```python
from build123d import *

# Parameters (mm, degrees)
F0_R     = 20
F1_DEPTH = 2
F2_W     = 370
F2_H     = 270
F3_DEPTH = 12


with BuildPart() as f1:
    # F0 (on Top) → F1 (new body)
    with BuildSketch(Plane.XY):
        with Locations((0, 200)):
            Circle(F0_R)
        with Locations((75, 200)):
            Circle(F0_R)
        with Locations((150, 200)):
            Circle(F0_R)
        with Locations((225, 200)):
            Circle(F0_R)
        with Locations((300, 200)):
            Circle(F0_R)
        with Locations((262.5, 150)):
            Circle(F0_R)
        with Locations((300, 100)):
            Circle(F0_R)
        with Locations((300, 0)):
            Circle(F0_R)
        with Locations((187.5, 150)):
            Circle(F0_R)
        with Locations((112.5, 150)):
            Circle(F0_R)
        with Locations((37.5, 150)):
            Circle(F0_R)
        with BuildLine():
            ThreePointArc((12, 84), (17.888544, 91.055728), (20, 100))
            ThreePointArc((20, 100), (-17.888544, 108.944272), (12, 84))
        make_face()
        with Locations((75, 100)):
            Circle(F0_R)
        with Locations((150, 100)):
            Circle(F0_R)
        with Locations((225, 100)):
            Circle(F0_R)
        with Locations((262.5, 50)):
            Circle(F0_R)
        with Locations((187.5, 50)):
            Circle(F0_R)
        with Locations((225, 0)):
            Circle(F0_R)
        with Locations((150, 0)):
            Circle(F0_R)
        with Locations((112.5, 50)):
            Circle(F0_R)
        with BuildLine():
            ThreePointArc((57.5, 50), (46.444272, 67.888544), (25.5, 66))
            Line((25.5, 66), (49.5, 34))
            ThreePointArc((49.5, 34), (55.388544, 41.055728), (57.5, 50))
        make_face()
        Circle(F0_R)
        with BuildLine():
            ThreePointArc((95, 0), (83.944272, 17.888544), (63, 16))
            ThreePointArc((63, 16), (66.055728, -17.888544), (95, 0))
        make_face()
        with BuildLine():
            Line((49.5, 34), (25.5, 66))
            ThreePointArc((25.5, 66), (21.5, 38), (49.5, 34))
        make_face()
    extrude(amount=-F1_DEPTH)


with BuildPart() as f3:
    # F2 (on Top) → F3 (new body)
    with BuildSketch(Plane.XY):
        with Locations((150, 100)):
            Rectangle(F2_W, F2_H)
    extrude(amount=-F3_DEPTH)

    # F4: cut F1
    add(f1.part, mode=Mode.SUBTRACT)


solid = f3.part
```
CAD build for the part. Positions are in the model's coordinates, mm. Round coordinates to 2 decimals unless told otherwise and drop trailing zeros. Loops run counter-clockwise (first coordinate to the right, second up) from the corner with the lowest first, then second, coordinate; pieces in that order, holes last. Notation, with made-up numbers: M 83.25,80.5 L 126.25,80.5 A23 ccw 126.25,111.5 Z; hole C 72.25,84 d1. An arc over 180 degrees is marked long. Use a Markdown table: item, result. Add a question column.
(1) Drill centre lines: line 1 (Y direction, x = 75, z = -0.5); line 2 (Y direction, x = 125, z = -1); line 3 (Z direction, x = 46, y = 133.5). Where is each one in solid material? Low to high.
(2) Pull direction Y, two halves, no side cores. Call faces 1 (the face through (300, 0, -2)), 2 (the face through (0, 100, -2)), 3 (the face through (147, 235, -6)): +Y half, -Y half, draft (parallel to the pull), parting line (faces both ways), or undercut.
(3) Cut at A-A (x = 300). Give the cut face in (y, z), and give its area (3 significant figures).
(4) Cut at B-B (y = 6). Give the cut face in (x, z).
(5) Cut at C-C (x = 37.5). Give the cut face in (y, z).
(6) Cut at D-D (y = 164). Give the cut face in (x, z).
(7) Flat gauge pins, fed straight in: pin 1 (20 mm diameter, centred on x = 9, y = 208.5, fed in from +Z); pin 2 (20 mm diameter, centred on x = 302.5, y = 96, fed in from +Z). Where does each tip first touch, or does it go through?
Geometry says:
| question | item | result |
|---|---|---|
| 1 | line 1 | y = -35 to -20, 20 to 80, 120 to 180, 220 to 235 |
| 1 | line 2 | y = -35 to 34.39, 65.61 to 134.39, 165.61 to 235 |
| 1 | line 3 | z = -12 to -2 |
| 2 | face 1 | undercut |
| 2 | face 2 | undercut |
| 2 | face 3 | +Y half |
| 3 | outline | M -35,-12 L 235,-12 L 235,0 L 220,0 L 220,-2 L 180,-2 L 180,0 L 120,0 L 120,-2 L 80,-2 L 80,0 L 20,0 L 20,-2 L -20,-2 L -20,0 L -35,0 Z |
| 3 | area | 3,000 mm² |
| 4 | outline | M -35,-12 L 335,-12 L 335,0 L 319.08,0 L 319.08,-2 L 280.92,-2 L 280.92,0 L 244.08,0 L 244.08,-2 L 205.92,-2 L 205.92,0 L 169.08,0 L 169.08,-2 L 130.92,-2 L 130.92,0 L 94.08,0 L 94.08,-2 L 55.92,-2 L 55.92,0 L 19.08,0 L 19.08,-2 L -19.08,-2 L -19.08,0 L -35,0 Z |
| 5 | outline | M -35,-12 L 235,-12 L 235,0 L 170,0 L 170,-2 L 130,-2 L 130,0 L 70,0 L 70,-2 L 30,-2 L 30,0 L -35,0 Z |
| 6 | outline | M -35,-12 L 335,-12 L 335,0 L 276.78,0 L 276.78,-2 L 248.22,-2 L 248.22,0 L 201.78,0 L 201.78,-2 L 173.22,-2 L 173.22,0 L 126.78,0 L 126.78,-2 L 98.22,-2 L 98.22,0 L 51.78,0 L 51.78,-2 L 23.22,-2 L 23.22,0 L -35,0 Z |
| 7 | pin 1 | stops at z = 0 |
| 7 | pin 2 | stops at z = -2 |
